Verification items for the finished model (mm, model axes). Give positions to 0.01 mm unless a question says otherwise; leave off trailing zeros. Loops run counter-clockwise (first coordinate to the right, second up) from the corner with the lowest first, then second, coordinate; pieces in that order, holes last. Notation, with made-up numbers: (84, -26) -> (118, -26) arc R27 cw to (118, -5) -> close; hole circle Ø10 at (-19.5, 71.5). An arc over 180 degrees is marked (long way). Use one line per item in the form item = value. Start each with the question number.
from build123d import *

# Parameters (mm, degrees)
SKETCH_1_W      = 10
SKETCH_1_H      = 10
SKETCH_1_R      = 2.1
EXTRUDE_1_DEPTH = 2
FILLET_1_R      = 2


with BuildPart() as part:
    # ｽｹｯﾁ1 → ﾎﾞｽ - 押し出し1 (new body)
    # profile 1 of 4: a face of its own
    with BuildSketch(Plane.XY):
        with Locations((0, 10)):
            Rectangle(SKETCH_1_W, SKETCH_1_H)
        with Locations((0, 10)):
            Circle(SKETCH_1_R, mode=Mode.SUBTRACT)
    # profile 2 of 4: a face of its own
    with BuildSketch(Plane.XY):
        Polygon((15, 5), (5, 15), (5, 5), align=None)
    # profile 3 of 4: a face of its own
    with BuildSketch(Plane.XY):
        Rectangle(SKETCH_1_W, SKETCH_1_H)
        Circle(SKETCH_1_R, mode=Mode.SUBTRACT)
    # profile 4 of 4: a face of its own
    with BuildSketch(Plane.XY):
        with Locations((10, 0)):
            Rectangle(SKETCH_1_W, SKETCH_1_H)
        with Locations((10, 0)):
            Circle(SKETCH_1_R, mode=Mode.SUBTRACT)
    extrude(amount=EXTRUDE_1_DEPTH)

    # ﾌｨﾚｯﾄ1
    fillet_1_edges = [part.edges().sort_by_distance(p)[0] for p in [
        (-5, -5, 1),
        (-5, 15, 1),
        (5, 15, 1),
        (15, 5, 1),
        (15, -5, 1),
    ]]
    fillet(fillet_1_edges, radius=FILLET_1_R)


solid = part.part
Item 1: Material ranges on line 1 (Y direction, x = 0, z = 1.2); line 2 (Y direction, x = 0.5, z = 1.4); line 3 (X direction, y = -1.5, z = 1.1), recorded low to high.
Item 2: Sectioned sample at C-C, the plane x = 0. Enter the section's corners in (y, z), and give its area (3 significant figures).
Item 3: Draft check along X on faces 1 (the flat face through (10, 10, 1)), 2 (the cylindrical face through (-4.4, 14.43, 1.01)), 3 (the cylindrical face through (-0.273, 12.082, 0.986)). Enter one of: +X half, -X half, draft (parallel to the pull), parting line (faces both ways), or undercut.
Item 4: Gauge pin test, flat ends, axial feed: pin 1 Ø2.5 at (x, y) = (10, 0) entering from -Z; pin 2 Ø5.5 at (x, y) = (0, 0) entering from +Z. Record the tip position at first contact, or that the pin passes through.
Item 5: Sectioned sample at A-A, the plane y = 10. Enter the section's corners in (x, z), and give its area (3 significant figures).
Item 6: Sectioned sample at B-B, the plane z = 0.4. Enter the section's corners in (x, y), and give its area (3 significant figures).
Outcome:
q1.line_1 = -5 to -2.1, 2.1 to 7.9, 12.1 to 15
q1.line_2 = -5 to -2.04, 2.04 to 7.96, 12.04 to 15
q1.line_3 = -5 to -1.47, 1.47 to 8.53, 11.47 to 15
q2.outline = (-5, 0) -> (-2.1, 0) -> (-2.1, 2) -> (-5, 2) -> close; (2.1, 0) -> (7.9, 0) -> (7.9, 2) -> (2.1, 2) -> close; (12.1, 0) -> (15, 0) -> (15, 2) -> (12.1, 2) -> close
q2.area = 23.2 mm^2
q3.face_1 = +X half
q3.face_2 = -X half
q3.face_3 = undercut
q4.pin_1 = through
q4.pin_2 = 2
q5.outline = (-5, 0) -> (-2.1, 0) -> (-2.1, 2) -> (-5, 2) -> close; (2.1, 0) -> (10, 0) -> (10, 2) -> (2.1, 2) -> close
q5.area = 21.6 mm^2
q6.outline = (-5, -3) arc R2 ccw to (-3, -5) -> (13, -5) arc R2 ccw to (15, -3) -> (15, 4.17) arc R2 ccw to (14.41, 5.59) -> (5.59, 14.41) arc R2 ccw to (4.17, 15) -> (-3, 15) arc R2 ccw to (-5, 13) -> close; hole circle Ø4.2 at (0, 0); hole circle Ø4.2 at (0, 10); hole circle Ø4.2 at (10, 0)
q6.area = 306 mm^2
